Here's how the part is built. I have some questions about the finished solid (model axes, mm). A direction names the side the tool comes from. Coordinates: 2 decimals unless noted, no trailing zeros. Write each loop counter-clockwise with the first axis right and the second up, starting at its lowest first coordinate (ties: lowest second). Pieces come first, ordered by that corner, then holes. Notation, with made-up numbers: M -28,-25.75 L -9,-25.75 A15 cw -9,-17.75 Z; hole C 66.5,1.5 d1. An arc over 180 degrees is marked long. Use a Markdown table: item, result.
```python
from build123d import *

# Parameters (mm, degrees)
BOX_W           = 28
BOX_H           = 30
BOX_DEPTH       = 5
SKETCH_W        = 3
SKETCH_H        = 30
SKETCH_W_2      = 7
PAD_DEPTH       = 24
SKETCH002_R     = 4.75
SKETCH002_W     = 1
SKETCH002_H     = 3
POCKET_DEPTH    = 4
POCKET001_DEPTH = 10
SKETCH003_W     = 5.5
SKETCH003_H     = 29
PAD001_DEPTH    = 4
SKETCH004_R     = 1.5
POCKET002_DEPTH = 5.3
POCKET003_DEPTH = 5


with BuildPart() as part:
    # Box → Box (new body)
    with BuildSketch(Plane.XY):
        with Locations((14, 15)):
            Rectangle(BOX_W, BOX_H)
    extrude(amount=BOX_DEPTH)

    # Sketch → Pad (new body)
    with BuildSketch(Plane.XY.offset(5)):
        with Locations((1.5, 15)):
            Rectangle(SKETCH_W, SKETCH_H)
        with Locations((24.5, 15)):
            Rectangle(SKETCH_W_2, SKETCH_H)
    extrude(amount=PAD_DEPTH)

    # Sketch002 → Pocket (cut, symmetric)
    with BuildSketch(Plane(origin=(0, 0, 0), x_dir=(0, -1, 0), z_dir=(-1, 0, 0))):
        with Locations((-12, 17)):
            Circle(SKETCH002_R)
        with Locations((-0.5, 17)):
            Rectangle(SKETCH002_W, SKETCH002_H)
    extrude(amount=POCKET_DEPTH, both=True, mode=Mode.SUBTRACT)

    # Sketch001 → Pocket001 (cut)
    with BuildSketch(Plane.YZ.offset(28)):
        with BuildLine():
            Line((19.827027, 22.20554), (19.827027, 11.79446))
            ThreePointArc((3.827027, 12.356455), (11.670031, 7.605793), (19.827027, 11.79446))
            Line((3.827027, 12.356455), (3.827027, 21.643545))
            ThreePointArc((19.827027, 22.20554), (11.670031, 26.394207), (3.827027, 21.643545))
        make_face()
    extrude(amount=-POCKET001_DEPTH, mode=Mode.SUBTRACT)

    # Sketch003 → Pad001 (new body)
    with BuildSketch(Plane(origin=(0, 0, 0), x_dir=(0, -1, 0), z_dir=(-1, 0, 0))):
        with Locations((-27.25, 14.5)):
            Rectangle(SKETCH003_W, SKETCH003_H)
    extrude(amount=PAD001_DEPTH)

    # Sketch004 → Pocket002 (cut)
    with BuildSketch(Plane(origin=(0, 30, 0), x_dir=(-1, 0, 0), z_dir=(0, 1, 0))):
        with Locations((-24.5, 10)):
            Circle(SKETCH004_R)
        with Locations((0.5, 10)):
            Circle(SKETCH004_R)
    extrude(amount=-POCKET002_DEPTH, mode=Mode.SUBTRACT)

    # Sketch005 → Pocket003 (cut)
    with BuildSketch(Plane.XY.offset(5)):
        with BuildLine():
            Line((21, 30), (3, 30))
            Line((3, 30), (3, 23))
            ThreePointArc((3, 23), (4.464466, 19.464466), (8, 18))
            Line((8, 18), (16, 18))
            ThreePointArc((16, 18), (19.535534, 19.464466), (21, 23))
            Line((21, 23), (21, 30))
        make_face()
    extrude(amount=-POCKET003_DEPTH, mode=Mode.SUBTRACT)


solid = part.part
```
1. Suppose I cut it at A-A on x = 24.5. Write out the boundary of the cut face in (y, z), and give its area (3 significant figures).
Answers follow:
| item | result |
|---|---|
| outline | M 0,0 L 30,0 L 30,8.5 L 24.7,8.5 L 24.7,11.5 L 30,11.5 L 30,29 L 0,29 Z; hole M 3.83,12.36 A9.4 ccw 19.83,11.79 L 19.83,22.21 A9.4 ccw 3.83,21.64 Z |
| area | 595 mm2 |
2. Which directions (+Z, -Z, +X, -X, +Y, -Y) give clear straight access to the entire face, cutting with the end or side of a thin tool? Please do faces 1 (the face through (-2, 24.5, 14)), 2 (the face through (19, 19, 3)), 3 (the face through (1.5, 0.5, 15.5)).
Answers follow:
| item | result |
|---|---|
| face 1 | +Z, -Z, -X, -Y |
| face 2 | +Z, -Z, +Y |
| face 3 | -X, -Y |
3. Suppose I cut it at B-B on z = 5.5. Write out the boundary of the cut face in (x, y).
Answers follow:
| item | result |
|---|---|
| outline | M -4,24.5 L 0,24.5 L 0,0 L 3,0 L 3,30 L -4,30 Z; M 21,0 L 28,0 L 28,30 L 21,30 Z |
4. We'd pull the mould along X, two halves only. Please class faces 4 (the face through (-0.175, 27.387, 8.536)), 5 (the face through (25, 3.827, 17)), 6 (the face through (0, 24.7, 10)), 7 (the face through (0, 12, 11)): +X half, -X half, draft (parallel to the pull), parting line (faces both ways), or undercut.
Answers follow:
| item | result |
|---|---|
| face 4 | undercut |
| face 5 | draft |
| face 6 | undercut |
| face 7 | -X half |
5. I need wall thicknesses on probe 1 along X at (y, z) = (27.25, 21); probe 2 along X at (y, z) = (20.5, 14.25); probe 3 along Z at (x, y) = (-0.5, 28.3). Which ranges of each line are inside material? Lowest first, please.
Answers follow:
| item | result |
|---|---|
| probe 1 | x = -4 to 3, 21 to 28 |
| probe 2 | x = 0 to 3, 21 to 28 |
| probe 3 | z = 0 to 8.5, 11.5 to 29 |
6. Will these pins go through, and if not, where does the flat tip stop? pin 1 Ø7.5 at (y, z) = (12, 17) entering from -X; pin 2 Ø10 at (x, z) = (10.5, 6.5) entering from +Y; pin 3 Ø7.5 at (y, z) = (16, 12) entering from -X; pin 4 Ø9 at (x, y) = (14, 15) entering from +Z.
Answers follow:
| item | result |
|---|---|
| pin 1 | passes through |
| pin 2 | stops at y = 18.54 |
| pin 3 | stops at x = 0 |
| pin 4 | stops at z = 5 |
7. Suppose I cut it at C-C on y = 9.5. Write out the boundary of the cut face in (x, z).
Answers follow:
| item | result |
|---|---|
| outline | M 0,0 L 28,0 L 28,7.94 L 21,7.94 L 21,5 L 3,5 L 3,12.96 L 0,12.96 Z; M 0,21.04 L 3,21.04 L 3,29 L 0,29 Z; M 21,26.06 L 28,26.06 L 28,29 L 21,29 Z |
8. Suppose I cut it at D-D on z = 23. Write out the boundary of the cut face in (x, y), and give its area (3 significant figures).
Answers follow:
| item | result |
|---|---|
| outline | M -4,24.5 L 0,24.5 L 0,0 L 3,0 L 3,30 L -4,30 Z; M 21,0 L 28,0 L 28,4.76 L 21,4.76 Z; M 21,19.24 L 28,19.24 L 28,30 L 21,30 Z |
| area | 221 mm2 |
